Read the model definition and answer for the solid it produces. Units are mm, in the model's axes. A direction names the side the tool comes from. Round coordinates to 2 decimals unless told otherwise and drop trailing zeros. Order: outer loops, then holes, each group sorted by start corner. A loop starts at its lowest first (then second) coordinate and runs counter-clockwise, first axis right, second up. Notation, with made-up numbers: (12.25, 30.5) -> (69.25, 30.5) arc R15 cw to (69.25, 42.5) -> close; hole circle Ø2 at (-1.5, 4). An arc over 180 degrees is marked (long way). Answer as a JSON object with one key per item and string values. Group by question number.
Item 1: The mould has two halves that part along X. Classify faces 1 (the cylindrical face through (31.2, 4.8, 4)), 2 (the flat face through (29, 0, -1)), 3 (the flat face through (20, -10, 3)): pulls with the +X half, pulls with the -X half, needs draft (parallel to the pull), parting line crosses it, or undercut.
Item 2: Section C-C, the plane z = 0.75 is taken. Write down the section's boundary in (x, y).
Item 3: Section B-B, the plane x = 6 is taken. Write down the section's boundary in (y, z).
Item 4: Consider probe 1 along Y at (x, z) = (32.7, 5); probe 2 along Z at (x, y) = (25, -4.75); probe 3 along Y at (x, z) = (6, 1.55). Determine where each line is inside the solid, lowest interval first. Write a range as from..to.
Item 5: Section A-A, the plane y = 0 is taken. Write down the section's boundary in (x, z).
Item 6: Section D-D, the plane x = 32 is taken. Write down the section's boundary in (y, z), plus the area to 3 significant figures.
Item 7: Given P1, Ø3.5, axis at x = 32.7, y = 4.75, coming from the -Z side; P2, Ø1.6, axis at y = 0.5, z = -1, coming from the -X side; P3, Ø0.8, axis at x = 17.5, z = -1, coming from the +Y side; P4, Ø2.5, axis at x = 32.7, y = -4.75, coming from the -Z side, each flat-ended and moving along its own axis, determine where each tip first touches the part or whether it passes through.
Item 8: For faces 4 (the flat face through (20, -2.25, -1)), 5 (the flat face through (20, 2.25, -1)), 6 (the flat face through (31, 5, 2)), determine the directions among +Z, -Z, +X, -X, +Y, -Y from which every point of the face is accessible in a straight line to the end or side of a thin tool.
from build123d import *

# Parameters (mm, degrees)
CROQUIS1_W              = 40
CROQUIS1_H              = 20
SALIENTE_EXTRUIR1_DEPTH = 6
CROQUIS2_W              = 18
CROQUIS2_H              = 4.5
SALIENTE_EXTRUIR2_DEPTH = 1.5
CROQUIS3_R              = 2.75
CORTAR_EXTRUIR1_DEPTH   = 8.5
CROQUIS4_R              = 1.5
CORTAR_EXTRUIR2_DEPTH   = 8.5
CORTAR_EXTRUIR3_DEPTH   = 2


with BuildPart() as part:
    # Croquis1 → Saliente-Extruir1 (new body)
    with BuildSketch(Plane.XY):
        with Locations((20, 0)):
            Rectangle(CROQUIS1_W, CROQUIS1_H)
    extrude(amount=SALIENTE_EXTRUIR1_DEPTH)

    # Croquis2 → Saliente-Extruir2 (add)
    with BuildSketch(Plane(origin=(0, 0, 0), x_dir=(-1, 0, 0), z_dir=(0, 0, -1))):
        with Locations((-20, 0)):
            Rectangle(CROQUIS2_W, CROQUIS2_H)
    extrude(amount=SALIENTE_EXTRUIR2_DEPTH)

    # Croquis3 → Cortar-Extruir1 (cut, through all)
    with BuildSketch(Plane.XY.offset(6)):
        with Locations((6, 0)):
            Circle(CROQUIS3_R)
    extrude(amount=-CORTAR_EXTRUIR1_DEPTH, mode=Mode.SUBTRACT)

    # Croquis4 → Cortar-Extruir2 (cut, through all)
    with BuildSketch(Plane.XY.offset(6)):
        with Locations((32.7, 4.75)):
            Circle(CROQUIS4_R)
        with Locations((32.7, -4.75)):
            Circle(CROQUIS4_R)
    extrude(amount=-CORTAR_EXTRUIR2_DEPTH, mode=Mode.SUBTRACT)

    # Croquis5 → Cortar-Extruir3 (cut)
    with BuildSketch(Plane(origin=(0, 0, 0), x_dir=(-1, 0, 0), z_dir=(0, 0, -1))):
        Polygon((-29.524573519, 4.75), (-31.11228676, 7.5), (-34.28771324, 7.5), (-35.875426481, 4.75), (-34.28771324, 2), (-31.11228676, 2), align=None)
        Polygon((-29.524573519, -4.75), (-31.11228676, -2), (-34.28771324, -2), (-35.875426481, -4.75), (-34.28771324, -7.5), (-31.11228676, -7.5), align=None)
    extrude(amount=-CORTAR_EXTRUIR3_DEPTH, mode=Mode.SUBTRACT)


solid = part.part
Values found:
{
 "1": {"face 1": "undercut", "face 2": "pulls with the +X half", "face 3": "needs draft"},
 "2": {"outline": "(0, -10) -> (40, -10) -> (40, 10) -> (0, 10) -> close; hole circle Ø5.5 at (6, 0); hole (29.52, -4.75) -> (31.11, -7.5) -> (34.29, -7.5) -> (35.88, -4.75) -> (34.29, -2) -> (31.11, -2) -> close; hole (29.52, 4.75) -> (31.11, 2) -> (34.29, 2) -> (35.88, 4.75) -> (34.29, 7.5) -> (31.11, 7.5) -> close"},
 "3": {"outline": "(-10, 0) -> (-2.75, 0) -> (-2.75, 6) -> (-10, 6) -> close; (2.75, 0) -> (10, 0) -> (10, 6) -> (2.75, 6) -> close"},
 "4": {"probe 1": "-10..-6.25, -3.25..3.25, 6.25..10", "probe 2": "0..6", "probe 3": "-10..-2.75, 2.75..10"},
 "5": {"outline": "(0, 0) -> (3.25, 0) -> (3.25, 6) -> (0, 6) -> close; (8.75, 0) -> (11, 0) -> (11, -1.5) -> (29, -1.5) -> (29, 0) -> (40, 0) -> (40, 6) -> (8.75, 6) -> close"},
 "6": {"outline": "(-10, 0) -> (-7.5, 0) -> (-7.5, 2) -> (-6.08, 2) -> (-6.08, 6) -> (-10, 6) -> close; (-3.42, 2) -> (-2, 2) -> (-2, 0) -> (2, 0) -> (2, 2) -> (3.42, 2) -> (3.42, 6) -> (-3.42, 6) -> close; (6.08, 2) -> (7.5, 2) -> (7.5, 0) -> (10, 0) -> (10, 6) -> (6.08, 6) -> close", "area": "76.8 mm2"},
 "7": {"P1": "z = 2", "P2": "x = 11", "P3": "y = 2.25", "P4": "through"},
 "8": {"face 4": "-Z, +X, -X, -Y", "face 5": "-Z, +X, -X, +Y", "face 6": "-Z"}
}
